Geometry: final body of the model. Coordinates: model frame, mm. Round coordinates to 2 decimals unless told otherwise and drop trailing zeros. Order: outer loops, then holes, each group sorted by start corner. A loop starts at its lowest first (then second) coordinate and runs counter-clockwise, first axis right, second up. Notation, with made-up numbers: (-13.75, 28.25) -> (29.25, 28.25) arc R11 cw to (29.25, 35.25) -> close; hole circle Ø2 at (44.5, -32.75). An arc over 180 degrees is marked (long way). Put each result on its own line as item: value.
```python
from build123d import *

# Parameters (mm, degrees)
F0_R     = 32.5
F0_R_2   = 30
F1_DEPTH = 20
F2_SIZE  = 0.5


with BuildPart() as f1:
    # F0 (on Front) → F1 (new body, symmetric)
    with BuildSketch(Plane.XZ):
        Circle(F0_R)
        Circle(F0_R_2, mode=Mode.SUBTRACT)
    extrude(amount=F1_DEPTH, both=True)

    # F2
    f2_edges = [f1.edges().sort_by_distance(p)[0] for p in [
        (-30, -20, 0),
        (30, 0, 0),
        (-30, 20, 0),
        (-32.5, 20, 0),
        (32.5, 0, 0),
        (-32.5, -20, 0),
    ]]
    chamfer(f2_edges, length=F2_SIZE)


solid = f1.part
```
1. Material intervals for probe 1 along Z at (x, y) = (0, -1); probe 2 along Z at (x, y) = (19.5, 2); probe 3 along X at (y, z) = (7.5, -9), sorted ascending.
Ans:
probe 1: -32.5 to -30, 30 to 32.5
probe 2: -26 to -22.8, 22.8 to 26
probe 3: -31.23 to -28.62, 28.62 to 31.23
2. Cut plane A-A on z = 0. Return loops of the section in (x, y), and give its area (3 significant figures).
Ans:
outline: (-32.5, -19.5) -> (-32, -20) -> (-30.5, -20) -> (-30, -19.5) -> (-30, 19.5) -> (-30.5, 20) -> (-32, 20) -> (-32.5, 19.5) -> close; (30, -19.5) -> (30.5, -20) -> (32, -20) -> (32.5, -19.5) -> (32.5, 19.5) -> (32, 20) -> (30.5, 20) -> (30, 19.5) -> close
area: 199 mm²
3. Cut plane B-B on x = 0. Return loops of the section in (y, z).
Ans:
outline: (-20, -32) -> (-19.5, -32.5) -> (19.5, -32.5) -> (20, -32) -> (20, -30.5) -> (19.5, -30) -> (-19.5, -30) -> (-20, -30.5) -> close; (-20, 30.5) -> (-19.5, 30) -> (19.5, 30) -> (20, 30.5) -> (20, 32) -> (19.5, 32.5) -> (-19.5, 32.5) -> (-20, 32) -> close
4. Draft query along X for faces 1 (the face through (-29.97, 0.27, 1.32)), 2 (the face through (31, -0.27, 9.76)), 3 (the face through (16.4, -20, -25.9)). Return one class per face: +X half, -X half, draft (parallel to the pull), parting line (faces both ways), or undercut.
Ans:
face 1: undercut
face 2: parting line
face 3: draft
5. Cut plane C-C on y = 12.5. Return loops of the section in (x, z).
Ans:
outline: circle Ø65 at (0, 0); hole circle Ø60 at (0, 0)
6. Contact query for flat-ended pins moving along their axis: P1, Ø8, axis at y = -4.5, z = 10.5, coming from the -X side; P2, Ø12, axis at x = 14.5, y = -13, coming from the -Z side; P3, Ø10, axis at x = -16, y = -3.5, coming from the +Z side; P4, Ø3, axis at x = -12.5, z = -25, coming from the -Y side (3 decimals). Output: stop coordinate, or through.
Ans:
P1: x = -31.84
P2: z = -31.37
P3: z = 30.58
P4: through
